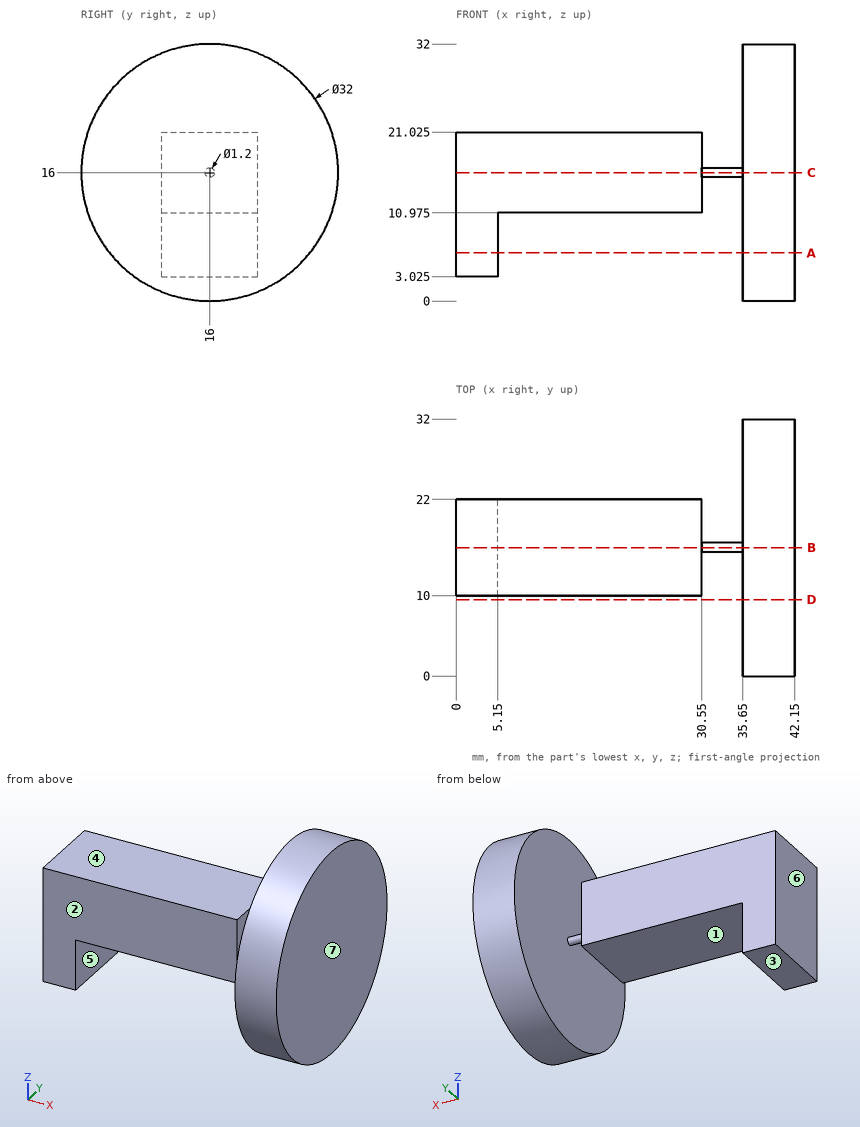
Source: three-view drawing plus pictorial views. Frame: mm from the lowest corner of the part. A direction names the side the tool comes from. Coordinates: 2 decimals unless noted, no trailing zeros. Loops run counter-clockwise (first coordinate to the right, second up) from the corner with the lowest first, then second, coordinate; pieces in that order, holes last. Notation, with made-up numbers: (-27, -39) - (17, -39) arc R22 cw to (17, -33) - close; hole circle Ø4 at (7.5, 12). An arc over 180 degrees is marked (long way). Answer in a Markdown table with one row per item. Add a question column.
Item 1: Contact query for flat-ended pins moving along their axis: P1, Ø3.5, axis at x = 16.5, y = 14.5, coming from the +Z side (3 decimals); P2, Ø9.5, axis at y = 24, z = 23, coming from the -X side; P3, Ø1, axis at y = 17, z = 23, coming from the -X side; P4, Ø14.5, axis at x = 14, z = 11, coming from the +Y side. Output: stop coordinate, or through.
Item 2: Mould query, pull axis X, two halves, no side actions, for the marked faces 4, 5, 6 and 7. Classes: released by +X, released by -X, zero draft, split by the parting line, or undercut.
Item 3: Section query C-C on z = 16. Return the cut outline in (x, y).
Item 4: Section query D-D on y = 9.5. Return the cut outline in (x, z).
Item 5: Section query A-A on z = 6. Return the cut outline in (x, y), then the cut area to 3 significant figures.
Item 6: Section query B-B on y = 16. Return the cut outline in (x, z) (3 decimals), then the cut area to 3 significant figures.
Item 7: Access query for the marked faces 1, 2 and 3. Directions: +Z, -Z, +X, -X, +Y, -Y. A direction counts if a zero-diameter tool reaches every point of the face in a straight line with its end or side. Return the directions, or none.
Item 8: Line query: line 1 along X through (y, z) = (28, 19); line 2 along Y through (x, z) = (5.5, 19); line 3 along Z through (x, y) = (30, 13.5) (3 decimals). Output: solid intervals per line, ascending. Write a range as [from, to].
Recorded:
| question | item | result |
|---|---|---|
| 1 | P1 | z = 21.025 |
| 1 | P2 | x = 0 |
| 1 | P3 | x = 35.65 |
| 1 | P4 | y = 22 |
| 2 | face 4 | zero draft |
| 2 | face 5 | undercut |
| 2 | face 6 | released by -X |
| 2 | face 7 | released by +X |
| 3 | outline | (0, 10) - (30.55, 10) - (30.55, 15.4) - (35.65, 15.4) - (35.65, 0) - (42.15, 0) - (42.15, 32) - (35.65, 32) - (35.65, 16.6) - (30.55, 16.6) - (30.55, 22) - (0, 22) - close |
| 4 | outline | (35.65, 1.38) - (42.15, 1.38) - (42.15, 30.62) - (35.65, 30.62) - close |
| 5 | outline | (0, 10) - (5.15, 10) - (5.15, 22) - (0, 22) - close; (35.65, 3.51) - (42.15, 3.51) - (42.15, 28.49) - (35.65, 28.49) - close |
| 5 | area | 224 mm^2 |
| 6 | outline | (0, 3.025) - (5.15, 3.025) - (5.15, 10.975) - (30.55, 10.975) - (30.55, 15.4) - (35.65, 15.4) - (35.65, 0) - (42.15, 0) - (42.15, 32) - (35.65, 32) - (35.65, 16.6) - (30.55, 16.6) - (30.55, 21.025) - (0, 21.025) - close |
| 6 | area | 562 mm^2 |
| 7 | face 1 | -Z, +Y, -Y |
| 7 | face 2 | +Z, -Z, -X, -Y |
| 7 | face 3 | -Z, -X, +Y, -Y |
| 8 | line 1 | [35.65, 42.15] |
| 8 | line 2 | [10, 22] |
| 8 | line 3 | [10.975, 21.025] |
